Part model, mm, in its own coordinate system. Face numbers are marked on the shaded views. A direction names the side the tool comes from. Round coordinates to 2 decimals unless told otherwise and drop trailing zeros. Write each loop counter-clockwise with the first axis right and the second up, starting at its lowest first coordinate (ties: lowest second). Pieces come first, ordered by that corner, then holes. Notation, with made-up numbers: M 9.25,76.25 L 61.25,76.25 A22 ccw 61.25,95.25 Z; hole C 50,-8 d4. An arc over 180 degrees is marked long. Use a Markdown table: item, result. Add a question column.
1) Slice it at D-D on z = 8. Write the cut outline in (x, y).
2) Drop flat-ended pins along their axis: P1, Ø5, axis at x = -5.66, y = 5.66, coming from the -Z side; P2, Ø3, axis at x = -1.5, z = 8, coming from the +Y side; P3, Ø1.5, axis at x = 6.5, z = 3.5, coming from the -Y side. Give the stop position or say it passes through.
3) Two-plate mould, pull along X, no slides. Class the marked faces 3, 4 and 5: released by +X, released by -X, zero draft, split by the parting line, or undercut.
4) Slice it at A-A on x = 0. Write the cut outline in (y, z), plus the area to 3 significant figures.
5) Wall check: probe 1 along Y at (x, z) = (0, 9.5); probe 2 along X at (y, z) = (-2, 13); probe 3 along Z at (x, y) = (-6.25, -8.75). Give the ranges that are in metal, low to high.
6) Which spindle directions (+Z, -Z, +X, -X, +Y, -Y) get a long thin tool onto all of the face, cutting with end or side? Do the marked faces 1 and 2. Say none if no direction does.
7) Slice it at C-C on x = -6.75. Write the cut outline in (y, z), plus the area to 3 significant figures.
```python
from build123d import *

# Parameters (mm, degrees)
SKETCH_R          = 11
PAD_DEPTH         = 3.5
SKETCH001_R       = 5
PAD001_DEPTH      = 10
PAD001_DEPTH_BACK = 4.5
SKETCH002_R       = 4
POCKET_DEPTH      = 14.501
SKETCH003_R       = 1.5
POCKET001_DEPTH   = 4.501


with BuildPart() as part:
    # Sketch → Pad (new body)
    with BuildSketch(Plane.XY):
        Circle(SKETCH_R)
    extrude(amount=PAD_DEPTH)

    # Sketch001 (on Face3 of Pad) → Pad001 (join, two sides)
    with BuildSketch(Plane.XY.offset(3.5)) as pad001_sk:
        Circle(SKETCH001_R)
    extrude(amount=PAD001_DEPTH)
    extrude(pad001_sk.sketch, amount=-PAD001_DEPTH_BACK)

    # Sketch002 (on Face7 of Pad001) → Pocket (cut, through all)
    with BuildSketch(Plane.XY.offset(13.5)):
        Circle(SKETCH002_R)
    extrude(amount=-POCKET_DEPTH, mode=Mode.SUBTRACT)

    # Sketch003 (on Face3 of Pocket) → Pocket001 (cut, through all)
    with BuildSketch(Plane.XY.offset(3.5)):
        with Locations((-5.656854, 5.656854)):
            Circle(SKETCH003_R)
        with Locations((5.656854, 5.656854)):
            Circle(SKETCH003_R)
        with Locations((5.656854, -5.656854)):
            Circle(SKETCH003_R)
        with Locations((-5.656854, -5.656854)):
            Circle(SKETCH003_R)
    extrude(amount=-POCKET001_DEPTH, mode=Mode.SUBTRACT)


solid = part.part
```
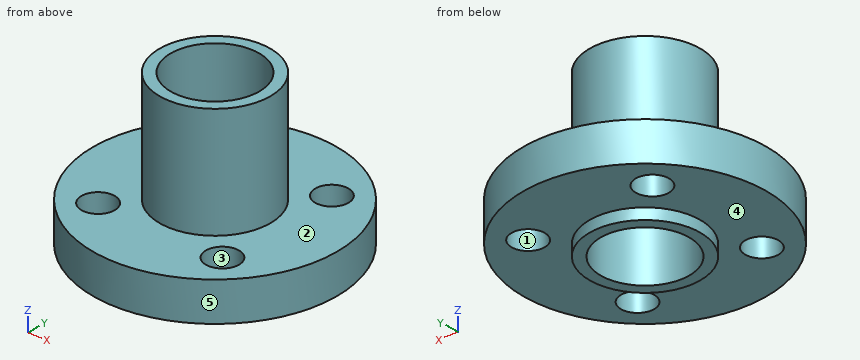
Entries:
| question | item | result |
|---|---|---|
| 1 | outline | C 0,0 d10; hole C 0,0 d8 |
| 2 | P1 | stops at z = 0 |
| 2 | P2 | stops at y = 5 |
| 2 | P3 | stops at y = -9.38 |
| 3 | face 3 | undercut |
| 3 | face 4 | zero draft |
| 3 | face 5 | split by the parting line |
| 4 | outline | M -11,0 L -5,0 L -5,-1 L -4,-1 L -4,13.5 L -5,13.5 L -5,3.5 L -11,3.5 Z; M 4,-1 L 5,-1 L 5,0 L 11,0 L 11,3.5 L 5,3.5 L 5,13.5 L 4,13.5 Z |
| 4 | area | 71.0 mm^2 |
| 5 | probe 1 | y = -5 to -4, 4 to 5 |
| 5 | probe 2 | x = -4.58 to -3.46, 3.46 to 4.58 |
| 5 | probe 3 | z = 0 to 3.5 |
| 6 | face 1 | +Z, -Z |
| 6 | face 2 | +Z |
| 7 | outline | M -8.69,0 L -6.68,0 L -6.68,3.5 L -8.69,3.5 Z; M -4.63,0 L 4.63,0 L 4.63,3.5 L -4.63,3.5 Z; M 6.68,0 L 8.69,0 L 8.69,3.5 L 6.68,3.5 Z |
| 7 | area | 46.4 mm^2 |
